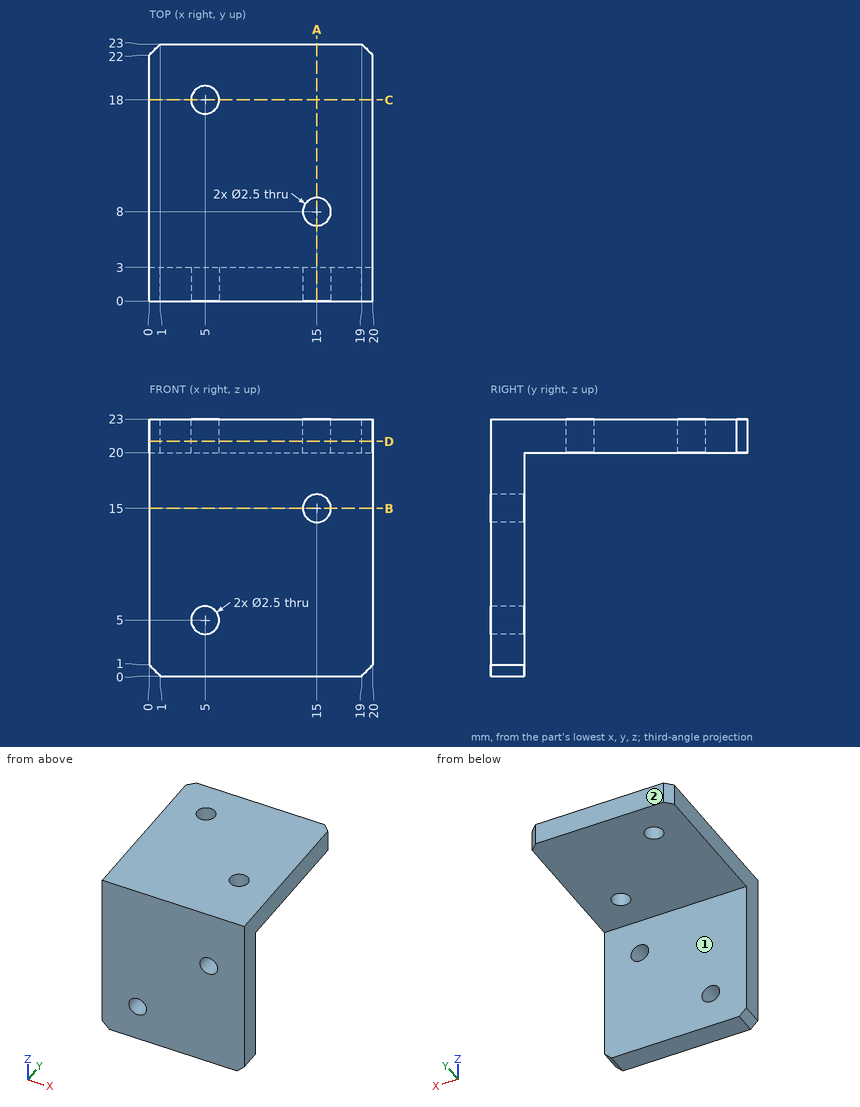
Input: dimensioned drawing with shaded views. Units: mm. Origin: part minimum x, y, z. A direction names the side the tool comes from. Round coordinates to 2 decimals unless told otherwise and drop trailing zeros. Order: outer loops, then holes, each group sorted by start corner. A loop starts at its lowest first (then second) coordinate and runs counter-clockwise, first axis right, second up.
Q1. Access query for the marked faces 1 and 2. Directions: +Z, -Z, +X, -X, +Y, -Y. A direction counts if a zero-diameter tool reaches every point of the face in a straight line with its end or side. Return the directions, or none.
Result sheet:
face 1: -Z, +X, -X, +Y
face 2: +Z, -Z, +X, -X, +Y
Q2. Section B-B, the plane z = 15. Output: boundary loops of the cut face in (x, y), and give its area (3 significant figures).
Result sheet:
outline: (0, 0) - (13.75, 0) - (13.75, 3) - (0, 3) - close; (16.25, 0) - (20, 0) - (20, 3) - (16.25, 3) - close
area: 52.5 mm2
Q3. Section A-A, the plane x = 15. Output: boundary loops of the cut face in (y, z), and give its area (3 significant figures).
Result sheet:
outline: (0, 0) - (3, 0) - (3, 13.75) - (0, 13.75) - close; (0, 16.25) - (3, 16.25) - (3, 20) - (6.75, 20) - (6.75, 23) - (0, 23) - close; (9.25, 20) - (23, 20) - (23, 23) - (9.25, 23) - close
area: 114 mm2
Q4. Pin query (flat end, axial travel): pin 1 (4 mm diameter, centred on x = 15, y = 8, fed in from -Z); pin 2 (6 mm diameter, centred on x = 15, z = 13.5, fed in from +Y). Return the tip coordinate at first contact, or that it passes through.
Result sheet:
pin 1: stops at z = 20
pin 2: stops at y = 3
Q5. Section D-D, the plane z = 21. Output: boundary loops of the cut face in (x, y), and give its area (3 significant figures).
Result sheet:
outline: (0, 0) - (20, 0) - (20, 22) - (19, 23) - (1, 23) - (0, 22) - close; hole circle Ø2.5 at (5, 18); hole circle Ø2.5 at (15, 8)
area: 449 mm2
Q6. Material intervals for probe 1 along X at (y, z) = (1.1, 5); probe 2 along Y at (x, z) = (5, 21.2); probe 3 along Y at (x, z) = (15, 20.7), sorted ascending.
Result sheet:
probe 1: x = 0 to 3.75, 6.25 to 20
probe 2: y = 0 to 16.75, 19.25 to 23
probe 3: y = 0 to 6.75, 9.25 to 23
Q7. Section C-C, the plane y = 18. Output: boundary loops of the cut face in (x, z), and give its area (3 significant figures).
Result sheet:
outline: (0, 20) - (3.75, 20) - (3.75, 23) - (0, 23) - close; (6.25, 20) - (20, 20) - (20, 23) - (6.25, 23) - close
area: 52.5 mm2
